Read the model definition and answer for the solid it produces. Units are mm, in the model's axes. Face numbers are marked on the shaded views. A direction names the side the tool comes from. Coordinates: 2 decimals unless noted, no trailing zeros. Order: outer loops, then holes, each group sorted by start corner. A loop starts at its lowest first (then second) coordinate and runs counter-clockwise, first axis right, second up. Notation, with made-up numbers: (82, 41.5) - (101, 41.5) arc R19 cw to (101, 71.5) - close; hole circle Ø11 at (51.5, 54.5). An arc over 180 degrees is marked (long way). Use one line per item in the form item = value.
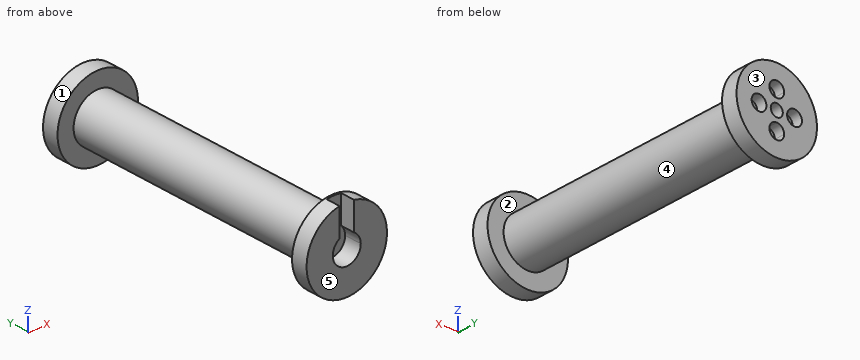
```python
from build123d import *

# Parameters (mm, degrees)
F0_R      = 9.525
F0_R_2    = 2.38125
F1_DEPTH  = 115.57
F2_R      = 15.875
F2_R_2    = 9.525
F3_DEPTH  = 6.35
F4_R      = 2.921
F5_DEPTH  = 4.064
F6_R      = 15.875
F6_R_2    = 9.525
F7_DEPTH  = 6.35
F8_W      = 5.715
F8_H      = 5.842
F9_DEPTH  = 34.4932
F11_DEPTH = 6.858


with BuildPart() as f1:
    # F0 (on Front) → F1 (new body)
    with BuildSketch(Plane.XZ):
        Circle(F0_R)
        Circle(F0_R_2, mode=Mode.SUBTRACT)
    extrude(amount=F1_DEPTH)

    # F2 (on face) → F3 (join)
    with BuildSketch(Plane(origin=(0, 0, 0), x_dir=(-1, 0, 0), z_dir=(0, 1, 0))):
        Circle(F2_R)
        Circle(F2_R_2, mode=Mode.SUBTRACT)
    extrude(amount=-F3_DEPTH)

    # F4 (on face) → F5 (cut)
    with BuildSketch(Plane(origin=(0, 0, 0), x_dir=(-1, 0, 0), z_dir=(0, 1, 0))):
        with BuildLine():
            ThreePointArc((2.921, 7), (-2.0654589078, 9.0654589078), (0, 4.079))
            ThreePointArc((0, 4.079), (2.0654589078, 4.9345410922), (2.921, 7))
        make_face()
        with Locations((-7, 0)):
            Circle(F4_R)
        with BuildLine():
            ThreePointArc((2.921, -7), (2.0654589078, -4.9345410922), (0, -4.079))
            ThreePointArc((0, -4.079), (-2.0654589078, -9.0654589078), (2.921, -7))
        make_face()
        with BuildLine():
            ThreePointArc((9.921, 0), (7, 2.921), (4.079, 0))
            ThreePointArc((4.079, 0), (7, -2.921), (9.921, 0))
        make_face()
    extrude(amount=-F5_DEPTH, mode=Mode.SUBTRACT)

    # F6 (on face) → F7 (join)
    with BuildSketch(Plane.XZ.offset(115.57)):
        Circle(F6_R)
        Circle(F6_R_2, mode=Mode.SUBTRACT)
    extrude(amount=-F7_DEPTH)

    # F8 (on Top) → F9 (cut)
    with BuildSketch(Plane.XY):
        with Locations((0, -112.8891035914)):
            Rectangle(F8_W, F8_H)
    extrude(amount=F9_DEPTH, mode=Mode.SUBTRACT)

    # F10 (on face) → F11 (cut)
    with BuildSketch(Plane.XZ.offset(115.57)):
        with BuildLine():
            Line((2.8575, 0), (2.8575, 4.7280856591))
            ThreePointArc((2.8575, 4.7280856591), (0, 5.5245), (-2.8575, 4.7280856591))
            Line((-2.8575, 4.7280856591), (-2.8575, 0))
            Line((-2.8575, 0), (-2.38125, 0))
            ThreePointArc((-2.38125, 0), (0, -2.38125), (2.38125, 0))
            Line((2.38125, 0), (2.8575, 0))
        make_face()
        with BuildLine():
            ThreePointArc((-2.8575, 4.7280856591), (-2.7142072047, -4.8117750883), (5.5245, 0))
            ThreePointArc((5.5245, 0), (4.8117750883, 2.7142072047), (2.8575, 4.7280856591))
            Line((2.8575, 4.7280856591), (2.8575, 0))
            Line((2.8575, 0), (2.38125, 0))
            ThreePointArc((2.38125, 0), (0, -2.38125), (-2.38125, 0))
            Line((-2.38125, 0), (-2.8575, 0))
            Line((-2.8575, 0), (-2.8575, 4.7280856591))
        make_face()
    extrude(amount=-F11_DEPTH, mode=Mode.SUBTRACT)


solid = f1.part
```
(1) Given pin 1 Ø4.5 at (x, z) = (0, 7) entering from +Y; pin 2 Ø8 at (y, z) = (-19, -0.5) entering from -X (3 decimals); pin 3 Ø1.7 at (y, z) = (-113, 7.5) entering from -X, each flat-ended and moving along its own axis, determine where each tip first touches the part or whether it passes through.
Answer list:
pin_1 = -4.06
pin_2 = -9.525
pin_3 = -14.42
(2) Section B-B, the plane x = 12.5 is taken. Write down the section's boundary in (y, z), then the cut area to 3 significant figures.
Answer list:
outline = (-115.57, -9.79) - (-109.22, -9.79) - (-109.22, 9.79) - (-115.57, 9.79) - close; (-6.35, -9.79) - (0, -9.79) - (0, 9.79) - (-6.35, 9.79) - close
area = 249 mm2
(3) Which of the six approach directions +Z, -Z, +X, -X, +Y, -Y give full straight-line access (tool end or side, diameter ignored) to the marked faces 4 and 5?
Answer list:
face_4 = none
face_5 = +Z, -Z, +X, -X, -Y
(4) Straight lines are drawn through the part: L1, parallel to Y at x = 13, z = 5.5; L2, parallel to X at y = -50, z = 0 (3 decimals). For each, find the intervals that lie inside material, in ascending order.
Answer list:
L1 = -115.57 to -109.22, -6.35 to 0
L2 = -9.525 to -2.381, 2.381 to 9.525
(5) The mould has two halves that part along Y. Classify the marked faces 1, 2 and 3: +Y half, -Y half, draft (parallel to the pull), parting line (faces both ways), or undercut.
Answer list:
face_1 = draft
face_2 = undercut
face_3 = +Y half
(6) Section D-D, the plane z = 13.5 is taken. Write down the section's boundary in (x, y), then the cut area to 3 significant figures.
Answer list:
outline = (-8.35, -115.57) - (-2.86, -115.57) - (-2.86, -109.97) - (2.86, -109.97) - (2.86, -115.57) - (8.35, -115.57) - (8.35, -109.22) - (-8.35, -109.22) - close; (-8.35, -6.35) - (8.35, -6.35) - (8.35, 0) - (-8.35, 0) - close
area = 180 mm2
(7) Section A-A, the plane z = -1 is taken. Write down the section's boundary in (x, y), then the cut area to 3 significant figures.
Answer list:
outline = (-15.84, -115.57) - (-5.43, -115.57) - (-5.43, -108.71) - (-2.16, -108.71) - (-2.16, 0) - (-4.26, 0) - (-4.26, -4.06) - (-9.74, -4.06) - (-9.74, 0) - (-15.84, 0) - (-15.84, -6.35) - (-9.47, -6.35) - (-9.47, -109.22) - (-15.84, -109.22) - close; (2.16, -108.71) - (5.43, -108.71) - (5.43, -115.57) - (15.84, -115.57) - (15.84, -109.22) - (9.47, -109.22) - (9.47, -6.35) - (15.84, -6.35) - (15.84, 0) - (9.74, 0) - (9.74, -4.06) - (4.26, -4.06) - (4.26, 0) - (2.16, 0) - close
area = 1,760 mm2
